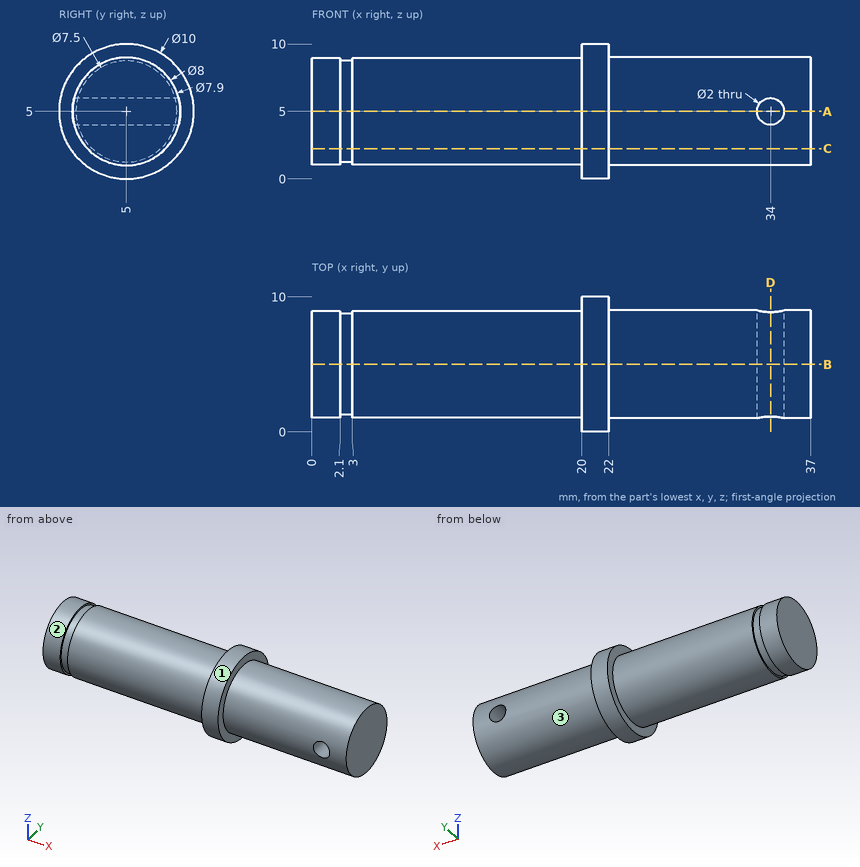
Job drawing, mm, ordinate dimensions from the low corner. One solid piece. A direction names the side the tool comes from. Round coordinates to 2 decimals unless told otherwise and drop trailing zeros. Order: outer loops, then holes, each group sorted by start corner. A loop starts at its lowest first (then second) coordinate and runs counter-clockwise, first axis right, second up. Notation, with made-up numbers: (4, 50.5) -> (40, 50.5) arc R11 ccw to (40, 70.5) -> close; hole circle Ø11 at (-34.75, -23). An arc over 180 degrees is marked (long way). Answer in a Markdown table with one row per item.
1) Wall check: L1, parallel to Z at x = 34, y = 5; L2, parallel to X at y = 3.5, z = 5; L3, parallel to X at y = 4.75, z = 5.5. Give the ranges that are in metal, low to high.
Values:
| item | result |
|---|---|
| L1 | 1 to 4, 6 to 9 |
| L2 | 0 to 33, 35 to 37 |
| L3 | 0 to 33.13, 34.87 to 37 |
2) Band-saw the part on C-C on z = 2.25. Give the cut face in (x, y).
Values:
| item | result |
|---|---|
| outline | (0, 2.16) -> (2.1, 2.16) -> (2.1, 2.45) -> (3, 2.45) -> (3, 2.16) -> (20, 2.16) -> (20, 0.82) -> (22, 0.82) -> (22, 2.1) -> (37, 2.1) -> (37, 7.9) -> (22, 7.9) -> (22, 9.18) -> (20, 9.18) -> (20, 7.84) -> (3, 7.84) -> (3, 7.55) -> (2.1, 7.55) -> (2.1, 7.84) -> (0, 7.84) -> close |
3) Which spindle directions (+Z, -Z, +X, -X, +Y, -Y) get a long thin tool onto all of the face, cutting with end or side? Do the marked faces 1, 2 and 3. Say none if no direction does.
Values:
| item | result |
|---|---|
| face 1 | +X, -X |
| face 2 | -X |
| face 3 | +X |
4) Band-saw the part on D-D on x = 34. Give the cut face in (y, z).
Values:
| item | result |
|---|---|
| outline | (1.13, 4) arc R4 ccw to (8.87, 4) -> close; (1.13, 6) -> (8.87, 6) arc R4 ccw to start |
5) Band-saw the part on A-A on z = 5. Give the cut face in (x, y), and give its area (3 significant figures).
Values:
| item | result |
|---|---|
| outline | (0, 1.05) -> (2.1, 1.05) -> (2.1, 1.25) -> (3, 1.25) -> (3, 1.05) -> (20, 1.05) -> (20, 0) -> (22, 0) -> (22, 1) -> (33, 1) -> (33, 9) -> (22, 9) -> (22, 10) -> (20, 10) -> (20, 8.95) -> (3, 8.95) -> (3, 8.75) -> (2.1, 8.75) -> (2.1, 8.95) -> (0, 8.95) -> close; (35, 1) -> (37, 1) -> (37, 9) -> (35, 9) -> close |
| area | 282 mm2 |
6) Pin check, flat tips, straight feed: P1, Ø2, axis at x = 4.5, z = 6.5, coming from the -Y side; P2, Ø5, axis at x = 30, z = 5.5, coming from the +Y side; P3, Ø5, axis at x = 30, y = 4, coming from the +Z side. Stop position of each tip, or through.
Values:
| item | result |
|---|---|
| P1 | y = 1.08 |
| P2 | y = 9 |
| P3 | z = 9 |
7) Band-saw the part on B-B on y = 5. Give the cut face in (x, z).
Values:
| item | result |
|---|---|
| outline | (0, 1.05) -> (2.1, 1.05) -> (2.1, 1.25) -> (3, 1.25) -> (3, 1.05) -> (20, 1.05) -> (20, 0) -> (22, 0) -> (22, 1) -> (37, 1) -> (37, 9) -> (22, 9) -> (22, 10) -> (20, 10) -> (20, 8.95) -> (3, 8.95) -> (3, 8.75) -> (2.1, 8.75) -> (2.1, 8.95) -> (0, 8.95) -> close; hole circle Ø2 at (34, 5) |
